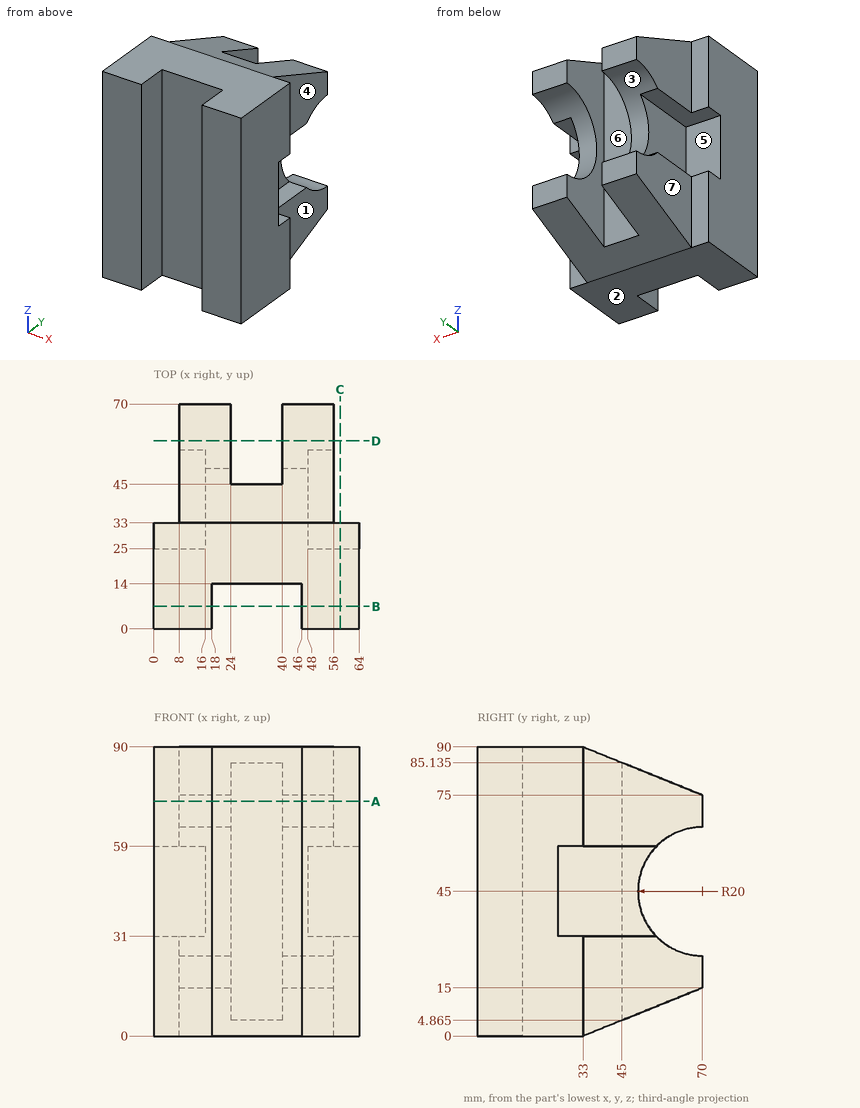
Job drawing, mm, ordinate dimensions from the low corner. One solid piece. A direction names the side the tool comes from. Round coordinates to 2 decimals unless told otherwise and drop trailing zeros. Loops run counter-clockwise (first coordinate to the right, second up) from the corner with the lowest first, then second, coordinate; pieces in that order, holes last. Notation, with made-up numbers: M 30,68 L 86,68 A18 ccw 86,82 Z; hole C 5.25,6.25 d7. An arc over 180 degrees is marked long. One line per question, with ' | ' between items. Start each with the question number.
Item 1: Wall check: line 1 (Z direction, x = 14.5, y = 26); line 2 (X direction, y = 13.5, z = 44.5); line 3 (X direction, y = 49, z = 82.5). Give the ranges that are in metal, low to high.
Item 2: Which spindle directions (+Z, -Z, +X, -X, +Y, -Y) get a long thin tool onto all of the face, cutting with end or side? Do the marked faces 4, 5, 6 and 7. Say none if no direction does.
Item 3: Cut at A-A, the plane z = 73. Write the cut outline in (x, y), plus the area to 3 significant figures.
Item 4: Cut at C-C, the plane x = 58. Write the cut outline in (y, z).
Item 5: Two-plate mould, pull along Z, no slides. Class the marked faces 1, 2 and 3: pulls with the +Z half, pulls with the -Z half, needs draft (parallel to the pull), parting line crosses it, or undercut.
Item 6: Cut at D-D, the plane y = 58.5. Write the cut outline in (x, z), plus the area to 3 significant figures.
Item 7: Cut at B-B, the plane y = 7. Write the cut outline in (x, z), plus the area to 3 significant figures.
Item 8: Pin check, flat tips, straight feed: pin 1 Ø8 at (x, y) = (34.5, 60) entering from +Z; pin 2 Ø17.5 at (x, y) = (58.5, 47) entering from -Z; pin 3 Ø9 at (x, z) = (2, 10) entering from +Y; pin 4 Ø13 at (x, z) = (34, 43) entering from +Y. Stop position of each tip, or through.
Responses:
1) line 1: z = 0 to 31, 59 to 90 | line 2: x = 0 to 18, 46 to 64 | line 3: x = 8 to 24, 40 to 56
2) face 4: +Z, -Z, +X, +Y | face 5: -X, +Y | face 6: +Z, -Z, +Y | face 7: +Z, -Z, -X, +Y
3) outline: M 0,0 L 18,0 L 18,14 L 46,14 L 46,0 L 64,0 L 64,33 L 56,33 L 56,70 L 40,70 L 40,45 L 24,45 L 24,70 L 8,70 L 8,33 L 0,33 Z | area: 3,100 mm²
4) outline: M 0,0 L 33,0 L 33,31 L 25,31 L 25,59 L 33,59 L 33,90 L 0,90 Z
5) face 1: needs draft | face 2: pulls with the -Z half | face 3: undercut
6) outline: M 8,10.34 L 24,10.34 L 24,28.64 L 8,28.64 Z; M 8,61.36 L 24,61.36 L 24,79.66 L 8,79.66 Z; M 40,10.34 L 56,10.34 L 56,28.64 L 40,28.64 Z; M 40,61.36 L 56,61.36 L 56,79.66 L 40,79.66 Z | area: 1,170 mm²
7) outline: M 0,0 L 18,0 L 18,90 L 0,90 Z; M 46,0 L 64,0 L 64,90 L 46,90 Z | area: 3,240 mm²
8) pin 1: passes through | pin 2: stops at z = 2.28 | pin 3: stops at y = 33 | pin 4: stops at y = 50.51
